from build123d import *

# Parameters (mm, degrees)
BOSS_EXTRUDE1_DEPTH = 16
BOSS_EXTRUDE2_DEPTH = 4
SKETCH3_R           = 2.1
CUT_EXTRUDE1_DEPTH  = 21
SKETCH4_R           = 4
CUT_EXTRUDE2_DEPTH  = 14
CUT_EXTRUDE3_DEPTH  = 3
CUT_EXTRUDE4_DEPTH  = 18


with BuildPart() as part:
    # Sketch1 → Boss-Extrude1 (new body)
    with BuildSketch(Plane.XY):
        with BuildLine():
            ThreePointArc((-15.884378154, 7.150884492), (-44.46319957, 12.91724959), (-38.696834472, -15.661571826))
            ThreePointArc((-38.696834472, -15.661571826), (-30.321063947, -1.224886034), (-15.884378154, 7.150884492))
        make_face()
    extrude(amount=BOSS_EXTRUDE1_DEPTH)

    # Sketch2 → Boss-Extrude2 (add)
    with BuildSketch(Plane(origin=(0, 0, 0), x_dir=(-1, 0, 0), z_dir=(0, 0, -1))):
        with BuildLine():
            ThreePointArc((8.160247818, 3.478149899), (-12.244043633, -43.789993613), (35.024099879, -23.385702162))
            ThreePointArc((35.024099879, -23.385702162), (36.287266145, -18.514575936), (39.968005835, -15.08301433))
            ThreePointArc((39.968005835, -15.08301433), (44.46319957, 12.91724959), (16.46293565, 8.422055855))
            ThreePointArc((16.46293565, 8.422055855), (13.031374044, 4.741316164), (8.160247818, 3.478149899))
        make_face()
    extrude(amount=BOSS_EXTRUDE2_DEPTH)

    # Sketch3 → Cut-Extrude1 (cut, through all)
    with BuildSketch(Plane(origin=(0, 0, -4), x_dir=(-1, 0, 0), z_dir=(0, 0, -1))):
        with Locations((40.220558883, -1.931992815)):
            Circle(SKETCH3_R)
        with Locations((29.613957165, 8.674608903)):
            Circle(SKETCH3_R)
    extrude(amount=-CUT_EXTRUDE1_DEPTH, mode=Mode.SUBTRACT)

    # Sketch4 → Cut-Extrude2 (cut)
    with BuildSketch(Plane(origin=(0, 0, -4), x_dir=(-1, 0, 0), z_dir=(0, 0, -1))):
        with Locations((40.220558883, -1.931992815)):
            Circle(SKETCH4_R)
        with Locations((29.613957165, 8.674608903)):
            Circle(SKETCH4_R)
    extrude(amount=-CUT_EXTRUDE2_DEPTH, mode=Mode.SUBTRACT)

    # Sketch5 → Cut-Extrude3 (cut)
    with BuildSketch(Plane(origin=(0, 0, -4), x_dir=(-1, 0, 0), z_dir=(0, 0, -1))):
        Polygon((23.603549525, -24.205856422), (7.340093558, -7.942400455), (-8.923362409, -24.205856422), (7.340093558, -40.46931239), align=None)
    extrude(amount=-CUT_EXTRUDE3_DEPTH, mode=Mode.SUBTRACT)

    # Sketch6 → Cut-Extrude4 (cut, through all)
    with BuildSketch(Plane(origin=(0, 0, -1), x_dir=(-1, 0, 0), z_dir=(0, 0, -1))):
        Polygon((7.340093558, -39.055098827), (22.189335963, -24.205856422), (7.340093558, -9.356614017), (-7.509148847, -24.205856422), align=None)
    extrude(amount=-CUT_EXTRUDE4_DEPTH, mode=Mode.SUBTRACT)


solid = part.part
Check sheet for the modelled part. Datum: model origin and axes. Units: mm. A direction names the side the tool comes from. Round coordinates to 2 decimals unless told otherwise and drop trailing zeros. Loops run counter-clockwise (first coordinate to the right, second up) from the corner with the lowest first, then second, coordinate; pieces in that order, holes last. Notation, with made-up numbers: M 21,-35.5 L 36,-35.5 A16 cw 36,-16.5 Z; hole C 51,41 d2. An arc over 180 degrees is marked long. One line per question, with ' | ' between items. Start each with the question number.
Item 1: Gauge pin test, flat ends, axial feed: pin 1 Ø18 at (x, y) = (-7, -13) entering from +Z; pin 2 Ø2.5 at (x, y) = (-41, -1.5) entering from -Z; pin 3 Ø5 at (x, z) = (-22.5, 6) entering from -Y. Record the tip position at first contact, or that the pin passes through.
Item 2: Section check B-B (y = -31). Record the boundary of the cut face in (x, z) (3 decimals).
Item 3: Scan lines: probe 1 along Z at (x, y) = (-20, 1.5); probe 2 along X at (y, z) = (0.5, -1); probe 3 along Y at (x, z) = (-10.5, -0.25). Record each from-to range of solid material in increasing order.
Item 4: Release check for a two-part mould opening along Y. For faces 4 (the face through (12.887, -43.125, -1.972)), 5 (the face through (0.68, -15.96, -2.52)), 6 (the face through (-30.488, -1.393, 7.888)), 7 (the face through (-22, -16, -4)) record: released by +Y, released by -Y, zero draft, split by the parting line, or undercut.
Item 5: Section check A-A (x = -18). Record the boundary of the cut face in (y, z).
Item 6: Set-up check for faces 1 (the face through (-43.9, -3.5, 2.9)), 2 (the face through (-16, -15, 0)), 3 (the face through (-14.869, -16.885, -0.507)): record each of +Z, -Z, +X, -X, +Y, -Y from which the full face is reachable in a straight line by a thin tool's end or side.
Item 7: Section check C-C (x = -10). Record the boundary of the cut face in (y, z).
Item 8: Section check D-D (y = -14). Record the boundary of the cut face in (x, z), and give its area (3 significant figures).
Worked out:
1) pin 1: z = 0 | pin 2: z = 10 | pin 3: y = 3.08
2) outline: M -34.19,-4 L -16.809,-4 L -16.809,-1 L -15.395,-1 L -15.395,0 L -34.19,0 Z; M 0.715,-1 L 2.129,-1 L 2.129,-4 L 19.51,-4 L 19.51,0 L 0.715,0 Z
3) probe 1: -4 to 0 | probe 2: -49.59 to -43.4, -37.04 to 5.18 | probe 3: -51.72 to -35.9, -12.52 to 3.72
4) face 4: split by the parting line | face 5: undercut | face 6: released by -Y | face 7: zero draft
5) outline: M -49.77,-4 L -29.81,-4 L -29.81,-1 L -28.4,-1 L -28.4,0 L -49.77,0 Z; M -20.02,-1 L -18.6,-1 L -18.6,-4 L 10.92,-4 L 10.92,16 L 6.5,16 L 6.5,0 L -20.02,0 Z
6) face 1: -Z | face 2: +Z, +X, -Y | face 3: +Z, -Z
7) outline: M -51.77,-4 L -37.81,-4 L -37.81,-1 L -36.4,-1 L -36.4,0 L -51.77,0 Z; M -12.02,-1 L -10.6,-1 L -10.6,-4 L 3.61,-4 L 3.61,0 L -12.02,0 Z
8) outline: M -41.82,-4 L -13.4,-4 L -13.4,-1 L -11.98,-1 L -11.98,0 L -38.2,0 L -38.2,16 L -41.82,16 Z; M -2.7,-1 L -1.28,-1 L -1.28,-4 L 18.41,-4 L 18.41,0 L -2.7,0 Z | area: 253 mm^2
